```python
from build123d import *

# Parameters (mm, degrees)
SKETCH1_W           = 56.017642274
SKETCH1_H           = 120.476854835
BOSS_EXTRUDE1_DEPTH = 22.907839
CUT_EXTRUDE1_DEPTH  = 56.017642


with BuildPart() as part:
    # Sketch1 → Boss-Extrude1 (new body)
    with BuildSketch(Plane.XY):
        with Locations((-45.790278616, -5.132568266)):
            Rectangle(SKETCH1_W, SKETCH1_H)
    extrude(amount=BOSS_EXTRUDE1_DEPTH)

    # Sketch2 → Cut-Extrude1 (cut)
    with BuildSketch(Plane(origin=(-17.781457479, 0, 0), x_dir=(0, 0, -1), z_dir=(1, 0, 0))):
        with BuildLine():
            ThreePointArc((-16.831723704, 19.373649849), (-14.292248498, 22.454133795), (-13.382838726, 26.341458007))
            Line((-13.382838726, 26.341458007), (-13.382838726, 55.105859152))
            Line((-13.382838726, 55.105859152), (-22.907838726, 55.105859152))
            Line((-22.907838726, 55.105859152), (-22.907838726, 10.40214091))
            ThreePointArc((-22.907838726, 10.40214091), (-21.998428954, 14.289465122), (-19.458953748, 17.369949068))
            Line((-19.458953748, 17.369949068), (-16.831723704, 19.373649849))
        make_face()
    extrude(amount=-CUT_EXTRUDE1_DEPTH, mode=Mode.SUBTRACT)


solid = part.part
```
Read the model definition and answer for the solid it produces. Units are mm, in the model's axes. A direction names the side the tool comes from. Round coordinates to 2 decimals unless told otherwise and drop trailing zeros. Write each loop counter-clockwise with the first axis right and the second up, starting at its lowest first coordinate (ties: lowest second). Pieces come first, ordered by that corner, then holes. Notation, with made-up numbers: (46, 65) -> (90, 65) arc R29 cw to (90, 88) -> close; hole circle Ø3 at (-4.75, -21.5). An arc over 180 degrees is marked (long way). Answer in a Markdown table with one row per item. Add a question column.
1) Find section C-C, the plane z = 15.5. Determine the outline of the cut face in (x, y).
2) Find section A-A, the plane x = -44. Determine the outline of the cut face in (y, z), and give its area (3 significant figures).
3) Which of the six approach directions +Z, -Z, +X, -X, +Y, -Y give full straight-line access (tool end or side, diameter ignored) to faces 1 (the face through (-46, -65.371, 11)), 2 (the face through (-45, 41, 13.383))?
4) Consider line 1 (Z direction, x = -54.5, y = 49.5); line 2 (Y direction, x = -56, z = 19); line 3 (Y direction, x = -41.5, z = 22). Determine where each line is inside the solid, lowest interval first.
5) Given P1, Ø1.5, axis at x = -61.5, y = 42, coming from the +Z side; P2, Ø8, axis at x = -66.5, z = 19.5, coming from the +Y side, each flat-ended and moving along its own axis, determine where each tip first touches the part or whether it passes through.
6) Find section B-B, the plane y = 16. Determine the outline of the cut face in (x, z).
Findings below:
| question | item | result |
|---|---|---|
| 1 | outline | (-73.8, -65.37) -> (-17.78, -65.37) -> (-17.78, 20.63) -> (-73.8, 20.63) -> close |
| 2 | outline | (-65.37, 0) -> (55.11, 0) -> (55.11, 13.38) -> (26.34, 13.38) arc R8.76 cw to (19.37, 16.83) -> (17.37, 19.46) arc R8.76 ccw to (10.4, 22.91) -> (-65.37, 22.91) -> close |
| 2 | area | 2,410 mm² |
| 3 | face 1 | +Z, -Z, +X, -X, -Y |
| 3 | face 2 | +Z, +X, -X, +Y |
| 4 | line 1 | 0 to 13.38 |
| 4 | line 2 | -65.37 to 17.72 |
| 4 | line 3 | -65.37 to 14.29 |
| 5 | P1 | z = 13.38 |
| 5 | P2 | y = 20.63 |
| 6 | outline | (-73.8, 0) -> (-17.78, 0) -> (-17.78, 20.89) -> (-73.8, 20.89) -> close |
